```python
from build123d import *

# Parameters (mm, degrees)
SKETCH1_R           = 0.3937
BOSS_EXTRUDE1_DEPTH = 1.6256


with BuildPart() as part:
    # Sketch1 → Boss-Extrude1 (new body)
    with BuildSketch(Plane(origin=(0, 0, 0), x_dir=(1, 0, 0), z_dir=(0, 1, 0))):
        Polygon((1.905, 1.4732), (17.54785055, 13.570337759), (19.05, 13.570337759), (19.05, 0), (1.905, 0), align=None)
        with Locations(Location((17.54785055, 11.562216741, 0), (0, 0, 270))):
            Circle(SKETCH1_R, mode=Mode.SUBTRACT)
        with Locations(Location((17.54785055, 9.276216741, 0), (0, 0, 270))):
            Circle(SKETCH1_R, mode=Mode.SUBTRACT)
        with Locations(Location((17.54785055, 6.990216741, 0), (0, 0, 270))):
            Circle(SKETCH1_R, mode=Mode.SUBTRACT)
        Polygon((5.577391241, 1.905), (16.002, 1.905), (16.002, 9.96669744), align=None, mode=Mode.SUBTRACT)
    extrude(amount=BOSS_EXTRUDE1_DEPTH)


solid = part.part
```
The model under review builds one solid part; all positions refer to its coordinate system, in mm. A direction names the side the tool comes from. Round coordinates to 2 decimals unless told otherwise and drop trailing zeros. Write each loop counter-clockwise with the first axis right and the second up, starting at its lowest first coordinate (ties: lowest second). Pieces come first, ordered by that corner, then holes. Notation, with made-up numbers: (-15.75, 11) - (7.25, 11) arc R37 cw to (7.25, 48) - close; hole circle Ø9 at (-15, 87). An arc over 180 degrees is marked (long way). Answer as CSV lines item,"result". Start each with the question number.
(1) We need section B-B on z = -2.75. State the section outline as (x, y) points, plus the area to 3 significant figures.
(2) For pin 1 Ø0.5 at (y, z) = (0.5, -5.5) entering from -X; pin 2 Ø5 at (x, z) = (13.5, -5.5) entering from -Y, all flat-tipped, find the tip position at first contact; note any pin that passes through.
(3) For faces 1 (the flat face through (11, 1, -1.905)), 2 (the flat face through (9.62, 0.8, -7.44)), list the 3-axis set-ups (+Z, -Z, +X, -X, +Y, -Y) from which the entire face can be reached by the end or side of a thin tool; tool diameter is ignored.
(4) To check wall thickness, follow line 1 (Z direction, x = 17.5, y = 1.2); line 2 (Z direction, x = 12, y = 0.9) (3 decimals); line 3 (Z direction, x = 14.75, y = 0.4) (3 decimals). State the ranges of each line that lie inside material, in increasing order.
(5) Draft analysis for pull direction Z (two halves, no side actions). For faces 3 (the flat face through (10.86, 0.8, -5.99)), 4 (the flat face through (11, 1, 0)), 5 (the flat face through (1.905, 1, -1)), 6 (the flat face through (16.002, 1, -6)), state which applies: pulls with the +Z half, pulls with the -Z half, needs draft (parallel to the pull), parting line crosses it, or undercut.
(6) We need section A-A on x = 6.5. State the section outline as (y, z) points (3 decimals), plus the area to 3 significant figures.
(7) We need section D-D on z = -7. State the section outline as (x, y) points, plus the area to 3 significant figures.
(8) We need section C-C on y = 0.25. State the section outline as (x, z) points (3 decimals).
Worked answers:
1,outline,"(3.56, 0) - (6.67, 0) - (6.67, 1.63) - (3.56, 1.63) - close; (16, 0) - (19.05, 0) - (19.05, 1.63) - (16, 1.63) - close"
1,area,"10.0 mm²"
2,pin 1,"x = 6.79"
2,pin 2,"y = 0"
3,face 1,"+Y, -Y"
3,face 2,"-Z, -X, +Y, -Y"
4,line 1,"-13.53 to -11.95, -11.17 to -9.67, -8.89 to -7.38, -6.6 to 0"
4,line 2,"-9.28 to -6.872, -1.905 to 0"
4,line 3,"-11.407 to -8.998, -1.905 to 0"
5,face 3,"undercut"
5,face 4,"pulls with the +Z half"
5,face 5,"needs draft"
5,face 6,"undercut"
6,outline,"(0, -5.027) - (1.626, -5.027) - (1.626, -2.618) - (0, -2.618) - close; (0, -1.905) - (1.626, -1.905) - (1.626, 0) - (0, 0) - close"
6,area,"7.01 mm²"
7,outline,"(9.05, 0) - (12.17, 0) - (12.17, 1.63) - (9.05, 1.63) - close; (16, 0) - (17.15, 0) - (17.15, 1.63) - (16, 1.63) - close; (17.94, 0) - (19.05, 0) - (19.05, 1.63) - (17.94, 1.63) - close"
7,area,"8.74 mm²"
8,outline,"(1.905, -1.473) - (17.548, -13.57) - (19.05, -13.57) - (19.05, 0) - (1.905, 0) - close; hole (5.577, -1.905) - (16.002, -9.967) - (16.002, -1.905) - close; hole circle Ø0.787 at (17.548, -11.562); hole circle Ø0.787 at (17.548, -9.276); hole circle Ø0.787 at (17.548, -6.99)"
